Verification items for the finished model (mm, model axes). Face numbers are marked on the shaded views. A direction names the side the tool comes from. Round coordinates to 2 decimals unless told otherwise and drop trailing zeros. Order: outer loops, then holes, each group sorted by start corner. A loop starts at its lowest first (then second) coordinate and runs counter-clockwise, first axis right, second up. Notation, with made-up numbers: M -25,-11 L 32,-11 A19 ccw 32,5 Z; hole C 73.25,55 d4. An arc over 180 degrees is marked long. One line per item, written item: value. Start each with the question number.
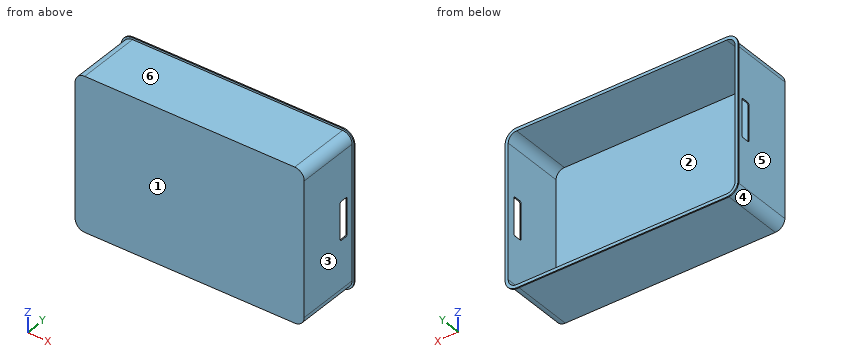
from build123d import *

# Parameters (mm, degrees)
SKETCH1_W               = 600
SKETCH1_H               = 400
BOSS_EXTRUDE1_DEPTH     = 170
FILLET1_R               = 25
SHELL1_T                = -3
EXTRUDE_THIN1_DEPTH     = 3
CUT_EXTRUDE2_DEPTH      = 1000
CUT_EXTRUDE2_DEPTH_BACK = 1000


with BuildPart() as part:
    # Sketch1 → Boss-Extrude1 (new body)
    with BuildSketch(Plane(origin=(0, 0, 0), x_dir=(1, 0, 0), z_dir=(0, 1, 0))):
        with Locations((300, 200)):
            Rectangle(SKETCH1_W, SKETCH1_H)
    extrude(amount=BOSS_EXTRUDE1_DEPTH)

    # Fillet1
    fillet1_edges = [part.edges().sort_by_distance(p)[0] for p in [
        (0, 85, -400),
        (600, 85, -400),
        (600, 85, 0),
        (0, 85, 0),
    ]]
    fillet(fillet1_edges, radius=FILLET1_R)

    # Shell1
    shell1_openings = [part.faces().sort_by_distance(p)[0] for p in [
        (300, 170, -200),
    ]]
    offset(amount=SHELL1_T, openings=shell1_openings, kind=Kind.INTERSECTION)

    # Sketch2 → Extrude-Thin1 (add)
    with BuildSketch(Plane(origin=(0, 170, 0), x_dir=(1, 0, 0), z_dir=(0, 1, 0))):
        with BuildLine():
            Line((-5, 25), (-5, 375))
            ThreePointArc((-5, 375), (3.786796564, 396.213203436), (25, 405))
            Line((25, 405), (575, 405))
            ThreePointArc((575, 405), (596.213203436, 396.213203436), (605, 375))
            Line((605, 375), (605, 25))
            ThreePointArc((605, 25), (596.213203436, 3.786796564), (575, -5))
            Line((575, -5), (25, -5))
            ThreePointArc((25, -5), (3.786796564, 3.786796564), (-5, 25))
        make_face()
        with BuildLine():
            Line((0, 25), (0, 375))
            ThreePointArc((0, 375), (7.32233047, 392.67766953), (25, 400))
            Line((25, 400), (575, 400))
            ThreePointArc((575, 400), (592.67766953, 392.67766953), (600, 375))
            Line((600, 375), (600, 25))
            ThreePointArc((600, 25), (592.67766953, 7.32233047), (575, 0))
            Line((575, 0), (25, 0))
            ThreePointArc((25, 0), (7.32233047, 7.32233047), (0, 25))
        make_face(mode=Mode.SUBTRACT)
    extrude(amount=-EXTRUDE_THIN1_DEPTH)

    # Sketch4 → Cut-Extrude2 (cut, two sides)
    with BuildSketch(Plane.ZY) as cut_extrude2_sk:
        with BuildLine():
            Line((-200, 150), (-155, 150))
            ThreePointArc((-155, 150), (-151.464466094, 148.535533906), (-150, 145))
            Line((-150, 145), (-150, 130))
            ThreePointArc((-150, 130), (-151.464466094, 126.464466094), (-155, 125))
            Line((-155, 125), (-245, 125))
            ThreePointArc((-245, 125), (-248.535533906, 126.464466094), (-250, 130))
            Line((-250, 130), (-250, 145))
            ThreePointArc((-250, 145), (-248.535533906, 148.535533906), (-245, 150))
            Line((-245, 150), (-200, 150))
        make_face()
    extrude(amount=CUT_EXTRUDE2_DEPTH, mode=Mode.SUBTRACT)
    extrude(cut_extrude2_sk.sketch, amount=-CUT_EXTRUDE2_DEPTH_BACK, mode=Mode.SUBTRACT)


solid = part.part
1. Tool access check on the marked faces 4, 5 and 6. Record the directions out of +Z, -Z, +X, -X, +Y, -Y that give a thin tool (end or side, any length) a straight path to the whole face; none if there is none.
2. Section check A-A (y = 136.5). Record the cut outline in (x, z).
3. Section check C-C (z = -232). Record the cut outline in (x, y), and give its area (3 significant figures).
4. Scan lines: line 1 along Z through (x, y) = (407.5, 129); line 2 along X through (y, z) = (135, -377.5); line 3 along X through (y, z) = (59, -278). Record each from-to range of solid material in increasing order.
5. Depth check by flat-ended pin: pin 1 (0.9 mm diameter, centred on x = 2, y = 134.5, fed in from -Z); pin 2 (10 mm diameter, centred on x = 332.5, y = 122, fed in from +Z); pin 3 (4 mm diameter, centred on x = 464.5, y = 22, fed in from -Z). Enter the tip coordinate at first touch or a pass-through.
6. Section check D-D (z = -120). Record the cut outline in (x, y), and give its area (3 significant figures).
7. Section check B-B (x = 427). Record the cut outline in (y, z).
8. Draft check along X on the marked faces 1, 2 and 3. Enter one of: released by +X, released by -X, zero draft, split by the parting line, or undercut.
Geometry check:
1. face 4: -Z, -X, -Y
1. face 5: +Z, -Z, -X, -Y
1. face 6: +Z, +X, -X, -Y
2. outline: M 0,-375 A25 ccw 25,-400 L 575,-400 A25 ccw 600,-375 L 600,-250 L 597,-250 L 597,-375 A22 cw 575,-397 L 25,-397 A22 cw 3,-375 L 3,-250 L 0,-250 Z; M 0,-150 L 3,-150 L 3,-25 A22 cw 25,-3 L 575,-3 A22 cw 597,-25 L 597,-150 L 600,-150 L 600,-25 A25 ccw 575,0 L 25,0 A25 ccw 0,-25 Z
3. outline: M -5,167 L 0,167 L 0,150 L 3,150 L 3,170 L -5,170 Z; M 0,0 L 600,0 L 600,125 L 597,125 L 597,3 L 3,3 L 3,125 L 0,125 Z; M 597,150 L 600,150 L 600,167 L 605,167 L 605,170 L 597,170 Z
3. area: 2,680 mm²
4. line 1: z = -400 to -397, -3 to 0
4. line 2: x = 0.13 to 3.14, 596.86 to 599.87
4. line 3: x = 0 to 3, 597 to 600
5. pin 1: stops at z = -385.79
5. pin 2: stops at z = 0
5. pin 3: stops at z = -400
6. outline: M -5,167 L 0,167 L 0,0 L 600,0 L 600,167 L 605,167 L 605,170 L 597,170 L 597,3 L 3,3 L 3,170 L -5,170 Z
6. area: 2,830 mm²
7. outline: M 0,-400 L 167,-400 L 167,-405 L 170,-405 L 170,-397 L 3,-397 L 3,-3 L 170,-3 L 170,5 L 167,5 L 167,0 L 0,0 Z
8. face 1: zero draft
8. face 2: undercut
8. face 3: released by +X
